```python
from build123d import *

# Parameters (mm, degrees)
SKETCH_R   = 53
SKETCH_R_2 = 2.5
PAD_DEPTH  = 5


with BuildPart() as part:
    # Sketch → Pad (new body)
    with BuildSketch(Plane.XY):
        Circle(SKETCH_R)
        Circle(SKETCH_R_2, mode=Mode.SUBTRACT)
    extrude(amount=PAD_DEPTH)

    # Sketch001 → Revolution (revolve)
    with BuildSketch(Plane.XZ):
        Polygon((53, 5), (47, 5), (47, 55), (48.75, 55), (48.75, 40), (51.25, 40), (51.25, 48), (53, 48), align=None)
    revolve(axis=Axis((0, 0, 0), (0, 0, 1)))


solid = part.part
```
Geometry check sheet. Reference: the model listing, model coordinates, mm. A direction names the side the tool comes from. Coordinates: 2 decimals unless noted, no trailing zeros. Order: outer loops, then holes, each group sorted by start corner. A loop starts at its lowest first (then second) coordinate and runs counter-clockwise, first axis right, second up.
Q1. Sectioned sample at C-C on z = 24. Record the cut outline in (x, y).
Reply:
outline: circle Ø106 at (0, 0); hole circle Ø94 at (0, 0)
Q2. Depth check by flat-ended pin: pin 1 Ø2 at (y, z) = (-34.5, 14) entering from +X; pin 2 Ø10 at (x, z) = (-12, 28.5) entering from +Y; pin 3 Ø2 at (y, z) = (-12.5, 17) entering from -X. Enter the tip coordinate at first touch or a pass-through.
Reply:
pin 1: stops at x = 41.07
pin 2: stops at y = 52.54
pin 3: stops at x = -51.74
Q3. Tool access check on faces 5 (the face through (26, 40, 55)), 6 (the face through (-1, -10, 5)). Record the directions out of +Z, -Z, +X, -X, +Y, -Y that give a thin tool (end or side, any length) a straight path to the whole face; none if there is none.
Reply:
face 5: +Z, +X, -X, +Y, -Y
face 6: +Z
Q4. Sectioned sample at A-A on y = 0. Record the cut outline in (x, z).
Reply:
outline: (-53, 0) - (-2.5, 0) - (-2.5, 5) - (-47, 5) - (-47, 55) - (-48.75, 55) - (-48.75, 40) - (-51.25, 40) - (-51.25, 48) - (-53, 48) - close; (2.5, 0) - (53, 0) - (53, 48) - (51.25, 48) - (51.25, 40) - (48.75, 40) - (48.75, 55) - (47, 55) - (47, 5) - (2.5, 5) - close
Q5. Sectioned sample at D-D on x = -31.5. Record the cut outline in (y, z), and give its area (3 significant figures).
Reply:
outline: (-42.62, 0) - (42.62, 0) - (42.62, 48) - (40.43, 48) - (40.43, 40) - (37.21, 40) - (37.21, 55) - (34.88, 55) - (34.88, 5) - (-34.88, 5) - (-34.88, 55) - (-37.21, 55) - (-37.21, 40) - (-40.43, 40) - (-40.43, 48) - (-42.62, 48) - close
area: 1,070 mm2
Q6. Draft check along X on faces 1 (the face through (-11.11, -50.03, 44.06)), 2 (the face through (28, 45, 24)), 3 (the face through (11, 1, 0)), 4 (the face through (-18.7, -45.3, 40)). Enter one of: released by +X, released by -X, zero draft, split by the parting line, or undercut.
Reply:
face 1: undercut
face 2: split by the parting line
face 3: zero draft
face 4: undercut
Q7. Thickness scan on probe 1 along Y at (x, z) = (0, 46.75); probe 2 along X at (y, z) = (1, 46.5); probe 3 along Y at (x, z) = (0, 24). Record the ranges inside material, lowest first.
Reply:
probe 1: y = -53 to -51.25, -48.75 to -47, 47 to 48.75, 51.25 to 53
probe 2: x = -52.99 to -51.24, -48.74 to -46.99, 46.99 to 48.74, 51.24 to 52.99
probe 3: y = -53 to -47, 47 to 53
